Here's how the part is built. I have some questions about the finished solid (model axes, mm). A direction names the side the tool comes from. Give positions to 0.01 mm unless a question says otherwise; leave off trailing zeros. Loops run counter-clockwise (first coordinate to the right, second up) from the corner with the lowest first, then second, coordinate; pieces in that order, holes last. Notation, with made-up numbers: (66.25, 57.25) - (72.25, 57.25) arc R26 ccw to (72.25, 74.25) - close; hole circle Ø5 at (61, 55). An arc over 180 degrees is marked (long way). Use a Markdown table: item, result.
from build123d import *

# Parameters (mm, degrees)
F0_W     = 127
F0_H     = 88.9
F1_DEPTH = 9.525
F3_W     = 101.6
F3_H     = 63.5
F4_DEPTH = 6.35
F5_R     = 9.525
F6_DEPTH = 127.001


with BuildPart() as f1:
    # F0 (on Top) → F1 (new body)
    with BuildSketch(Plane.XY):
        with Locations((-63.5, -44.45)):
            Rectangle(F0_W, F0_H)
    extrude(amount=-F1_DEPTH)

    # F3 (on face) → F4 (cut)
    with BuildSketch(Plane.XY):
        with Locations((-63.5, -44.45)):
            Rectangle(F3_W, F3_H)
    extrude(amount=-F4_DEPTH, mode=Mode.SUBTRACT)

    # F5
    f5_edges = [f1.edges().sort_by_distance(p)[0] for p in [
        (-12.7, -12.7, -3.175),
        (-114.3, -12.7, -3.175),
        (-114.3, -76.2, -3.175),
        (-12.7, -76.2, -3.175),
    ]]
    fillet(f5_edges, radius=F5_R)

    # F2 (on face) → F6 (cut, through all)
    with BuildSketch(Plane(origin=(-127, 0, 0), x_dir=(0, -1, 0), z_dir=(-1, 0, 0))):
        Polygon((88.9, 0), (0, 0), (88.9, -6.35), align=None)
    extrude(amount=-F6_DEPTH, mode=Mode.SUBTRACT)


solid = f1.part
(1) On a 3-axis mill with a long thin cutter (end or side, diameter ignored), from which of +Z, -Z, +X, -X, +Y, -Y can I reach the whole of each face in a straight line? I mean faces 5 (the face through (-64, -44, -9.525)), 6 (the face through (-12.7, -40, -4)). Say none if no direction works.
A:
| item | result |
|---|---|
| face 5 | -Z, +X, -X, +Y, -Y |
| face 6 | +Z |
(2) Will these pins go through, and if not, where does the flat tip stop? pin 1 (1 mm diameter, centred on y = -52, z = -2, fed in from -X); pin 2 (6 mm diameter, centred on x = -37.5, y = -43.5, fed in from +Z); pin 3 (1.5 mm diameter, centred on x = -49.5, z = -7, fed in from +Y).
A:
| item | result |
|---|---|
| pin 1 | through |
| pin 2 | z = -6.35 |
| pin 3 | y = 0 |
(3) We'd pull the mould along X, two halves only. Please class faces 1 (the face through (0, -35, -6)), 2 (the face through (-64, -88.9, -8)), 3 (the face through (-114.3, -40, -4)), 4 (the face through (-127, -35, -6)): pulls with the +X half, pulls with the -X half, needs draft (parallel to the pull), parting line crosses it, or undercut.
A:
| item | result |
|---|---|
| face 1 | pulls with the +X half |
| face 2 | needs draft |
| face 3 | undercut |
| face 4 | pulls with the -X half |
(4) If I drill on line 1 (X direction, y = -28.5, z = -3.25); line 2 (Z direction, x = -46.5, y = -55) (3 decimals); line 3 (Y direction, x = -86, z = -4), over which ranges is the centre line in solid material (lowest first)?
A:
| item | result |
|---|---|
| line 1 | -127 to -114.3, -12.7 to 0 |
| line 2 | -9.525 to -6.35 |
| line 3 | -12.7 to 0 |
(5) Suppose I cut it at A-A on x = -63.5. Write out the boundary of the cut face in (y, z) (3 decimals), plus the area to 3 significant figures.
A:
| item | result |
|---|---|
| outline | (-88.9, -9.525) - (0, -9.525) - (0, 0) - (-12.7, -0.907) - (-12.7, -6.35) - (-76.2, -6.35) - (-76.2, -5.443) - (-88.9, -6.35) - close |
| area | 363 mm2 |
